Model file for the job. Use its own axes, mm. A direction names the side the tool comes from. Give positions to 0.01 mm unless a question says otherwise; leave off trailing zeros. Write each loop counter-clockwise with the first axis right and the second up, starting at its lowest first coordinate (ties: lowest second). Pieces come first, ordered by that corner, then holes.
```python
from build123d import *

# Parameters (mm, degrees)
F0_W     = 102.0282506943
F0_H     = 102.0282581449
F1_DEPTH = 101.6
F2_R     = 25.4
F3_DEPTH = 101.6
F6_W     = 50.8
F6_H     = 50.8
F7_DEPTH = 130.048
F8_R     = 6.35


with BuildPart() as f1:
    # F0 (on Top) → F1 (new body)
    with BuildSketch(Plane.XY):
        Rectangle(F0_W, F0_H)
    extrude(amount=F1_DEPTH)

    # F2 (on face) → F3 (join)
    with BuildSketch(Plane.XY.offset(101.6)):
        Circle(F2_R)
    extrude(amount=F3_DEPTH)

    # F4 (on face) → F5 (revolve)
    with BuildSketch(Plane.XY.offset(203.2)):
        with BuildLine():
            Line((0, -25.4), (0, -38.1))
            ThreePointArc((0, -38.1), (38.1, 0), (0, 38.1))
            Line((0, 38.1), (0, 25.4))
            ThreePointArc((0, 25.4), (17.9605122421, 17.9605122421), (25.4, 0))
            ThreePointArc((25.4, 0), (17.9605122421, -17.9605122421), (0, -25.4))
        make_face()
        with BuildLine():
            ThreePointArc((0, 25.4), (-25.4, 0), (0, -25.4))
            Line((0, -25.4), (0, 0))
            Line((0, 0), (0, 25.4))
        make_face()
    revolve(axis=Axis((0, 0, 203.2), (0, -1, 0)))

    # F6 (on face) → F7 (cut)
    with BuildSketch(Plane.XZ.offset(51.0141290724)):
        with Locations((0, 50.8)):
            Rectangle(F6_W, F6_H)
    extrude(amount=-F7_DEPTH, mode=Mode.SUBTRACT)

    # F8
    f8_edges = [f1.edges().sort_by_distance(p)[0] for p in [
        (51.014125, 0, 101.6),
        (51.014125, -51.014129, 50.8),
        (51.014125, 0, 0),
        (51.014125, 51.014129, 50.8),
        (0, -51.014129, 101.6),
        (0, -51.014129, 0),
        (-51.014125, -51.014129, 50.8),
        (-51.014125, 0, 101.6),
        (0, 51.014129, 101.6),
        (-51.014125, 51.014129, 50.8),
        (0, 51.014129, 0),
        (-51.014125, 0, 0),
        (-25.4, 0, 101.6),
        (-25.4, 0, 174.801937),
    ]]
    fillet(f8_edges, radius=F8_R)


solid = f1.part
```
1. Pull direction X, two halves, no side cores. Call faces 4 (the flat face through (-1, 51.014, 80)), 5 (the cylindrical face through (-49.203, 49.105, 51.422)), 6 (the flat face through (25.4, -1, 50)): +X half, -X half, draft (parallel to the pull), parting line (faces both ways), or undercut.
Calculated:
face 4: draft
face 5: -X half
face 6: undercut
2. Which spindle directions (+Z, -Z, +X, -X, +Y, -Y) get a long thin tool onto all of the face, cutting with end or side? Do faces 1 (the flat face through (-30, 11, 101.6)), 2 (the cylindrical face through (0.625, 49.105, 99.789)), 3 (the flat face through (0, -1, 76.2)). Say none if no direction does.
Calculated:
face 1: none
face 2: +Z, +X, -X, +Y
face 3: +Y, -Y
3. Slice it at B-B, the plane z = 188. Write the cut outline in (x, y), and give its area (3 significant figures).
Calculated:
outline: circle Ø69.87 at (0, 0)
area: 3,830 mm2
4. Probe probe 1 along Z at (x, y) = (-18, -29); probe 2 along Z at (x, y) = (-5, 27); probe 3 along X at (y, z) = (-44, 53). List the from-to ranges inside material, lowest first.
Calculated:
probe 1: z = 0 to 25.4, 76.2 to 101.6, 186.27 to 220.13
probe 2: z = 0 to 25.4, 76.2 to 103.27, 176.79 to 229.61
probe 3: x = -51.01 to -25.4, 25.4 to 51.01
5. Pin check, flat tips, straight feed: P1, Ø12, axis at x = 36, z = 122, coming from the +Y side; P2, Ø10, axis at x = -27.5, z = 169, coming from the +Y side; P3, Ø12, axis at x = 13, y = -31.5, coming from the +Z side; P4, Ø6, axis at x = 30.5, y = 30, coming from the +Z side. Stop position of each tip, or through.
Calculated:
P1: passes through
P2: stops at y = 11.79
P3: stops at z = 228.95
P4: stops at z = 101.6
6. Slice it at A-A, the plane x = -40.5. Write the cut outline in (y, z), and give its area (3 significant figures).
Calculated:
outline: (-51.01, 6.35) arc R6.35 ccw to (-44.66, 0) - (44.66, 0) arc R6.35 ccw to (51.01, 6.35) - (51.01, 95.25) arc R6.35 ccw to (44.66, 101.6) - (-44.66, 101.6) arc R6.35 ccw to (-51.01, 95.25) - close
area: 10,300 mm2
